CAD build for the part. Positions are in the model's coordinates, mm. Face numbers are marked on the shaded views. A direction names the side the tool comes from. Coordinates: 2 decimals unless noted, no trailing zeros. Order: outer loops, then holes, each group sorted by start corner. A loop starts at its lowest first (then second) coordinate and runs counter-clockwise, first axis right, second up. Notation, with made-up numbers: M -12,28 L 36,28 A23 ccw 36,62 Z; hole C 69,65 d6. An arc over 180 degrees is marked long. One line per item, written item: value.
from build123d import *

# Parameters (mm, degrees)
BASPROSKE_W         = 6
BASPROSKE_H         = 16.5
TOOTHCUT_DEPTH      = 25.093567606
TEETHCUTS_COUNT     = 20
TEETHCUTS_ANGLE     = 342
BORSKE_R            = 2
BORE_DEPTH          = 50.0000508
SKETCH1_W           = 14.532002023
SKETCH1_H           = 35.225661126
CUT_EXTRUDE1_DEPTH  = 5
SKETCH3_W           = 7
SKETCH3_H           = 90
BOSS_EXTRUDE2_DEPTH = 3
SKETCH4_W           = 10
SKETCH4_H           = 30
BOSS_EXTRUDE3_DEPTH = 4
FILLET1_R           = 10
FILLET4_R           = 5
FILLET5_R           = 1
CUT_EXTRUDE4_DEPTH  = 4
CUT_EXTRUDE6_DEPTH  = 4
FILLET6_R           = 5


with BuildPart() as part:
    # BasProSke → Base-Revolve (revolve)
    with BuildSketch(Plane(origin=(0, 0, 0), x_dir=(1, 0, 0), z_dir=(0, 1, 0)), mode=Mode.PRIVATE) as base_revolve_sk:
        with Locations((3, 8.25)):
            Rectangle(BASPROSKE_W, BASPROSKE_H)
    revolve(base_revolve_sk.sketch.rotate(Axis((-10, 0, 0), (1, 0, 0)), 180), axis=Axis((-10, 0, 0), (1, 0, 0)))

    # TooCutSke → ToothCut (cut, through all)
    with BuildSketch(Plane(origin=(0, 0, 0), x_dir=(0, 0, -1), z_dir=(1, 0, 0))):
        with BuildLine():
            ThreePointArc((0.74381438, 13.102904875), (0, 13.124), (-0.74381438, 13.102904875))
            ThreePointArc((-0.74381438, 13.102904875), (-1.226473103, 14.852072512), (-2.209965745, 16.376962373))
            ThreePointArc((-2.209965745, 16.376962373), (0, 16.5254), (2.209965745, 16.376962373))
            ThreePointArc((2.209965745, 16.376962373), (1.226473103, 14.852072512), (0.74381438, 13.102904875))
        make_face()
    toothcut = extrude(amount=TOOTHCUT_DEPTH, mode=Mode.SUBTRACT)

    # TeethCuts: ToothCut ×20 about axis
    teethcuts_axis = Axis((-10, 0, 0), (1, 0, 0))
    for i in range(1, TEETHCUTS_COUNT):
        add(toothcut.rotate(teethcuts_axis, i * TEETHCUTS_ANGLE / (TEETHCUTS_COUNT - 1)), mode=Mode.SUBTRACT)

    # BorSke → Bore (cut, symmetric)
    with BuildSketch(Plane(origin=(0, 0, 0), x_dir=(0, 0, -1), z_dir=(1, 0, 0))):
        with Locations(Location((0, 0, 0), (0, 0, 180))):
            Circle(BORSKE_R)
    extrude(amount=BORE_DEPTH, both=True, mode=Mode.SUBTRACT)

    # Sketch1 → Cut-Extrude1 (cut, symmetric)
    with BuildSketch(Plane(origin=(3, 0, 0), x_dir=(0, 0, -1), z_dir=(1, 0, 0))):
        with Locations((-10.60761178, 0.822467031)):
            Rectangle(SKETCH1_W, SKETCH1_H)
    extrude(amount=CUT_EXTRUDE1_DEPTH, both=True, mode=Mode.SUBTRACT)

    # Sketch3 → Boss-Extrude2 (add, symmetric)
    with BuildSketch(Plane(origin=(3, 0, 0), x_dir=(0, 0, -1), z_dir=(1, 0, 0))):
        with Locations((-6.841610769, 29.963142125)):
            Rectangle(SKETCH3_W, SKETCH3_H)
    extrude(amount=BOSS_EXTRUDE2_DEPTH, both=True)

    # Sketch4 → Boss-Extrude3 (add, symmetric)
    with BuildSketch(Plane(origin=(3, 0, 0), x_dir=(0, 0, -1), z_dir=(1, 0, 0))):
        with Locations((-5.341610769, 59.963142125)):
            Rectangle(SKETCH4_W, SKETCH4_H)
    extrude(amount=BOSS_EXTRUDE3_DEPTH, both=True)

    # Fillet1
    # the kernel refuses this fillet: 10 mm, written as the material it takes off along each edge
    with BuildSketch(Plane(origin=(29.848480035, -15.036857875, 10.341610769), x_dir=(0, 0, -1), z_dir=(-1, 0, 0))) as fillet1_piece_1:
        with BuildLine():
            CenterArc((10, -9.539392014), FILLET1_R, 107.457603124, 72.542396876)
            Line((0, -9.539392014), (-0.2, -9.539392014))
            Line((-0.2, -9.539392014), (-0.2, 0))
            Line((-0.2, 0), (0, 0.2))
            ThreePointArc((0, 0.2), (3.5, 0.2), (6.94, 0.19078784))
            Line((6.94, 0.19078784), (7, 0))
        make_face()
    extrude(amount=53.696960071, mode=Mode.SUBTRACT)

    # Fillet4
    # the kernel refuses this fillet: 5 mm, written as the material it takes off along each edge
    with BuildSketch(Plane(origin=(19.5, 44.963142125, 0.341610769), x_dir=(0, 0, 1), z_dir=(-1, 0, 0))) as fillet4_piece_1_section:
        with BuildLine():
            CenterArc((FILLET4_R, FILLET4_R), FILLET4_R, 180, 90)
            Line((0, FILLET4_R), (0, 0))
            Line((0, 0), (FILLET4_R, 0))
        make_face()
    fillet4_piece_1 = extrude(amount=33, mode=Mode.PRIVATE)
    fillet4_piece_1 = split(fillet4_piece_1, bisect_by=Plane(origin=(12.75, 45.013801365, 3.341610769), z_dir=(0, 0, 1)), keep=Keep.TOP, mode=Mode.PRIVATE)
    fillet4_piece_1 = split(fillet4_piece_1, bisect_by=Plane(origin=(6, 45.013801365, 4.050354099), z_dir=(1, 0, 0)), keep=Keep.TOP, mode=Mode.PRIVATE)
    add(fillet4_piece_1, mode=Mode.SUBTRACT)
    with BuildSketch(Plane(origin=(19.5, 44.963142125, 0.341610769), x_dir=(0, 0, 1), z_dir=(-1, 0, 0))) as fillet4_piece_2_section:
        with BuildLine():
            CenterArc((FILLET4_R, FILLET4_R), FILLET4_R, 180, 90)
            Line((0, FILLET4_R), (0, 0))
            Line((0, 0), (FILLET4_R, 0))
        make_face()
    fillet4_piece_2 = extrude(amount=33, mode=Mode.PRIVATE)
    fillet4_piece_2 = split(fillet4_piece_2, bisect_by=Plane(origin=(12.75, 46.181868003, 3.341610769), z_dir=(0, 0, -1)), keep=Keep.TOP, mode=Mode.PRIVATE)
    fillet4_piece_2 = split(fillet4_piece_2, bisect_by=Plane(origin=(6, 46.181868003, 1.266861087), z_dir=(1, 0, 0)), keep=Keep.TOP, mode=Mode.PRIVATE)
    add(fillet4_piece_2, mode=Mode.SUBTRACT)
    with BuildSketch(Plane(origin=(19.5, 44.963142125, 0.341610769), x_dir=(0, 0, 1), z_dir=(-1, 0, 0))) as fillet4_piece_3_section:
        with BuildLine():
            CenterArc((FILLET4_R, FILLET4_R), FILLET4_R, 180, 90)
            Line((0, FILLET4_R), (0, 0))
            Line((0, 0), (FILLET4_R, 0))
        make_face()
    fillet4_piece_3 = extrude(amount=33, mode=Mode.PRIVATE)
    fillet4_piece_3 = split(fillet4_piece_3, bisect_by=Plane(origin=(0, 46.181868003, 1.266861087), z_dir=(1, 0, 0)), keep=Keep.TOP, mode=Mode.PRIVATE)
    fillet4_piece_3 = split(fillet4_piece_3, bisect_by=Plane(origin=(3, 46.181868003, 3.341610769), z_dir=(0, 0, -1)), keep=Keep.TOP, mode=Mode.PRIVATE)
    fillet4_piece_3 = split(fillet4_piece_3, bisect_by=Plane(origin=(6, 46.181868003, 1.266861087), z_dir=(-1, 0, 0)), keep=Keep.TOP, mode=Mode.PRIVATE)
    add(fillet4_piece_3, mode=Mode.SUBTRACT)
    with BuildSketch(Plane(origin=(19.5, 44.963142125, 0.341610769), x_dir=(0, 0, 1), z_dir=(-1, 0, 0))) as fillet4_piece_4_section:
        with BuildLine():
            CenterArc((FILLET4_R, FILLET4_R), FILLET4_R, 180, 90)
            Line((0, FILLET4_R), (0, 0))
            Line((0, 0), (FILLET4_R, 0))
        make_face()
    fillet4_piece_4 = extrude(amount=33, mode=Mode.PRIVATE)
    fillet4_piece_4 = split(fillet4_piece_4, bisect_by=Plane(origin=(0, 45.013801365, 4.050354099), z_dir=(-1, 0, 0)), keep=Keep.TOP, mode=Mode.PRIVATE)
    fillet4_piece_4 = split(fillet4_piece_4, bisect_by=Plane(origin=(-6.75, 45.013801365, 3.341610769), z_dir=(0, 0, 1)), keep=Keep.TOP, mode=Mode.PRIVATE)
    add(fillet4_piece_4, mode=Mode.SUBTRACT)
    with BuildSketch(Plane(origin=(19.5, 44.963142125, 0.341610769), x_dir=(0, 0, 1), z_dir=(-1, 0, 0))) as fillet4_piece_5_section:
        with BuildLine():
            CenterArc((FILLET4_R, FILLET4_R), FILLET4_R, 180, 90)
            Line((0, FILLET4_R), (0, 0))
            Line((0, 0), (FILLET4_R, 0))
        make_face()
    fillet4_piece_5 = extrude(amount=33, mode=Mode.PRIVATE)
    fillet4_piece_5 = split(fillet4_piece_5, bisect_by=Plane(origin=(0, 46.181868003, 1.266861087), z_dir=(-1, 0, 0)), keep=Keep.TOP, mode=Mode.PRIVATE)
    fillet4_piece_5 = split(fillet4_piece_5, bisect_by=Plane(origin=(-6.75, 46.181868003, 3.341610769), z_dir=(0, 0, -1)), keep=Keep.TOP, mode=Mode.PRIVATE)
    add(fillet4_piece_5, mode=Mode.SUBTRACT)
    with BuildSketch(Plane(origin=(19.5, 74.963142125, 10.341610769), x_dir=(0, -1, 0), z_dir=(-1, 0, 0))) as fillet4_piece_6:
        with BuildLine():
            CenterArc((FILLET4_R, -FILLET4_R), FILLET4_R, 90, 90)
            Line((0, -FILLET4_R), (0, 0))
            Line((0, 0), (FILLET4_R, 0))
        make_face()
    extrude(amount=33, mode=Mode.SUBTRACT)
    with BuildSketch(Plane(origin=(19.5, 74.963142125, 0.341610769), x_dir=(0, -1, 0), z_dir=(-1, 0, 0))) as fillet4_piece_7:
        with BuildLine():
            CenterArc((FILLET4_R, FILLET4_R), FILLET4_R, 180, 90)
            Line((0, FILLET4_R), (0, 0))
            Line((0, 0), (FILLET4_R, 0))
        make_face()
    extrude(amount=33, mode=Mode.SUBTRACT)

    # Fillet5
    fillet5_edges = [part.edges().sort_by_distance(p)[0] for p in [
        (3, 45.38056643, 3.341610769),
    ]]
    fillet(fillet5_edges, radius=FILLET5_R)

    # Sketch5 → Cut-Extrude4 (cut, symmetric)
    with BuildSketch(Plane(origin=(3, 0, 0), x_dir=(0, 0, -1), z_dir=(1, 0, 0))):
        Polygon((-0.646757919, 13.233276671), (-0.74381438, 13.102904875), (-3.341610769, 15.036857875), (-3.193884675, 16.241167121), (-1.325890901, 16.884807614), align=None)
    extrude(amount=CUT_EXTRUDE4_DEPTH, both=True, mode=Mode.SUBTRACT)

    # Sketch7 → Cut-Extrude6 (cut, symmetric)
    with BuildSketch(Plane(origin=(3, 0, 0), x_dir=(0, 0, -1), z_dir=(1, 0, 0))):
        Polygon((-7.363012022, -15.230284447), (-8.903180744, -10.664623645), (7.578586785, -11.037675843), (10.397777633, -17.422865984), (-4.980223066, -17.422865984), align=None)
    extrude(amount=CUT_EXTRUDE6_DEPTH, both=True, mode=Mode.SUBTRACT)

    # Fillet6
    fillet6_edges = [part.edges().sort_by_distance(p)[0] for p in [
        (3, -10.664623645, 8.903180744),
    ]]
    fillet(fillet6_edges, radius=FILLET6_R)


solid = part.part
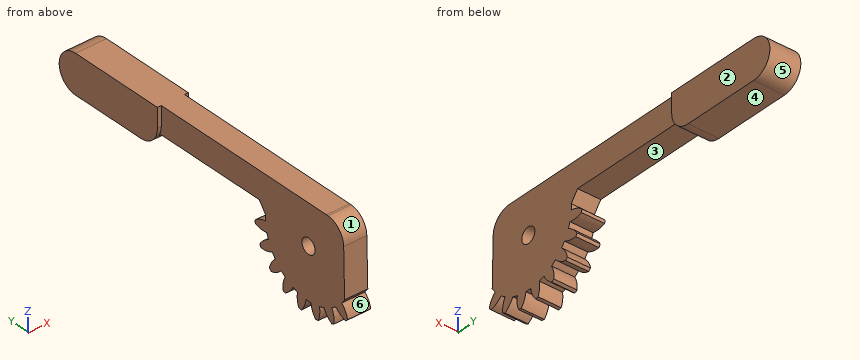
Q1. Slice it at C-C (y = 65). List the corners of the cut face in (x, z), plus the area to 3 significant figures.
Recorded:
outline: M -1,0.34 L 7,0.34 L 7,10.34 L -1,10.34 Z
area: 80.0 mm^2
Q2. Which spindle directions (+Z, -Z, +X, -X, +Y, -Y) get a long thin tool onto all of the face, cutting with end or side? Do the marked faces 4, 5 and 6. Say none if no direction does.
Recorded:
face 4: -Z, +X, -X, +Y
face 5: +X, -X, +Y
face 6: +X, -X, -Y
Q3. Slice it at B-B (z = 7). List the corners of the cut face in (x, y), plus the area to 3 significant figures.
Recorded:
outline: M -1,44.96 L 0,44.96 L 0,-10.46 L 6,-10.46 L 6,44.96 L 7,44.96 L 7,74.68 L -1,74.68 Z
area: 570 mm^2
Q4. Pin check, flat tips, straight feed: pin 1 Ø8 at (y, z) = (12.5, -6) entering from +X; pin 2 Ø10 at (y, z) = (18, 1) entering from -X; pin 3 Ø1.5 at (x, z) = (0, -10) entering from +Y. Stop position of each tip, or through.
Recorded:
pin 1: stops at x = 6
pin 2: stops at x = 0
pin 3: stops at y = 11.76
Q5. Slice it at A-A (y = 0). List the corners of the cut face in (x, z), plus the area to 3 significant figures.
Recorded:
outline: M 0,-13.12 L 6,-13.12 L 6,-2 L 0,-2 Z; M 0,2 L 6,2 L 6,10.34 L 0,10.34 Z
area: 117 mm^2
Q6. Drill centre lines: line 1 along Y through (x, z) = (5.25, -13.5); line 2 along X through (y, z) = (1, -2.5); line 3 along Y through (x, z) = (1.65, 0). Where is each one in solid material? Low to high.
Recorded:
line 1: y = -7.85 to -5.55, -3.45 to -0.8, 0.8 to 3.45, 5.55 to 7.85
line 2: x = 0 to 6
line 3: y = -10.87 to -2, 2 to 13.12
Q7. Mould opens along Y. For the marked faces 1, 2 and 3 say: released by +Y, released by -Y, zero draft, split by the parting line, or undercut.
Recorded:
face 1: released by -Y
face 2: zero draft
face 3: undercut
